Input: part model. Units: mm. Frame: model coordinates. Face numbers are marked on the shaded views. A direction names the side the tool comes from. Give positions to 0.01 mm unless a question says otherwise; leave off trailing zeros. Loops run counter-clockwise (first coordinate to the right, second up) from the corner with the lowest first, then second, coordinate; pieces in that order, holes last. Notation, with made-up numbers: (-32, -25.5) - (10, -25.5) arc R32 cw to (10, 0.5) - close; hole circle Ø5 at (51.25, -22.75). An arc over 180 degrees is marked (long way). Answer as a JSON object with one key per item and string values.
from build123d import *

# Parameters (mm, degrees)
SKETCH1_W           = 26.35
SKETCH1_H           = 50
SKETCH1_W_2         = 20
SKETCH1_H_2         = 43.65
BOSS_EXTRUDE1_DEPTH = 35
SKETCH2_W           = 26.35
SKETCH2_H           = 50
BOSS_EXTRUDE2_DEPTH = 3.175
BOSS_EXTRUDE3_DEPTH = 5
FILLET1_R           = 4
SKETCH6_W           = 10
SKETCH6_H           = 5
CUT_EXTRUDE3_DEPTH  = 3.175
SKETCH8_R           = 3.05
CUT_EXTRUDE5_DEPTH  = 2.7
BOSS_EXTRUDE4_START = -3.175
SKETCH9_W           = 6
SKETCH9_H           = 4
BOSS_EXTRUDE4_DEPTH = 12.5
SKETCH10_R          = 1
CUT_EXTRUDE6_DEPTH  = 15.675


with BuildPart() as part:
    # Sketch1 → Boss-Extrude1 (new body)
    with BuildSketch(Plane(origin=(0, 0, 0), x_dir=(1, 0, 0), z_dir=(0, 1, 0))):
        Rectangle(SKETCH1_W, SKETCH1_H)
        Rectangle(SKETCH1_W_2, SKETCH1_H_2, mode=Mode.SUBTRACT)
    extrude(amount=BOSS_EXTRUDE1_DEPTH)

    # Sketch2 → Boss-Extrude2 (add)
    with BuildSketch(Plane(origin=(0, 35, 0), x_dir=(1, 0, 0), z_dir=(0, 1, 0))):
        Rectangle(SKETCH2_W, SKETCH2_H)
    extrude(amount=BOSS_EXTRUDE2_DEPTH)

    # Sketch4 → Boss-Extrude3 (add)
    with BuildSketch(Plane.XZ):
        with BuildLine():
            Line((-8.6, -20), (-8.6, -21.825))
            Line((-8.6, -21.825), (-1.4, -21.825))
            Line((-1.4, -21.825), (-1.4, -20))
            ThreePointArc((-1.4, -20), (-5, -16.4), (-8.6, -20))
        make_face()
        with BuildLine():
            Line((-8.6, 21.825), (-1.4, 21.825))
            Line((-1.4, 21.825), (-1.4, 20))
            ThreePointArc((-1.4, 20), (-5, 16.4), (-8.6, 20))
            Line((-8.6, 20), (-8.6, 21.825))
        make_face()
    extrude(amount=-BOSS_EXTRUDE3_DEPTH)

    # Fillet1
    fillet1_edges = [part.edges().sort_by_distance(p)[0] for p in [
        (-13.175, 38.175, 0),
        (0, 38.175, 25),
        (13.175, 38.175, 0),
        (0, 38.175, -25),
        (13.175, 19.0875, 25),
        (-13.175, 19.0875, 25),
        (-13.175, 19.0875, -25),
        (13.175, 19.0875, -25),
    ]]
    fillet(fillet1_edges, radius=FILLET1_R)

    # Sketch6 → Cut-Extrude3 (cut)
    with BuildSketch(Plane.ZY.offset(13.175)):
        with Locations((0, 20.675)):
            Rectangle(SKETCH6_W, SKETCH6_H)
    extrude(amount=-CUT_EXTRUDE3_DEPTH, mode=Mode.SUBTRACT)

    # Sketch8 → Cut-Extrude5 (cut)
    with BuildSketch(Plane.XZ):
        with Locations(Location((-5, -20, 0), (0, 0, 270))):
            Circle(SKETCH8_R)
        with Locations(Location((-5, 20, 0), (0, 0, 270))):
            Circle(SKETCH8_R)
    extrude(amount=-CUT_EXTRUDE5_DEPTH, mode=Mode.SUBTRACT)

    # Sketch9 → Boss-Extrude4 (add)
    with BuildSketch(Plane(origin=(13.175, 0, 0), x_dir=(0, 0, -1), z_dir=(1, 0, 0)).offset(BOSS_EXTRUDE4_START)):
        with Locations((19.5, 9.6)):
            Rectangle(SKETCH9_W, SKETCH9_H)
        with Locations((-9.25, 9.6)):
            Rectangle(SKETCH9_W, SKETCH9_H)
    extrude(amount=-BOSS_EXTRUDE4_DEPTH)

    # Sketch10 → Cut-Extrude6 (cut)
    with BuildSketch(Plane.XZ.offset(-7.6)):
        with Locations(Location((3.75, 8.575, 0), (0, 0, 270))):
            Circle(SKETCH10_R)
        with Locations(Location((3.75, -18.825, 0), (0, 0, 270))):
            Circle(SKETCH10_R)
    extrude(amount=-CUT_EXTRUDE6_DEPTH, mode=Mode.SUBTRACT)


solid = part.part
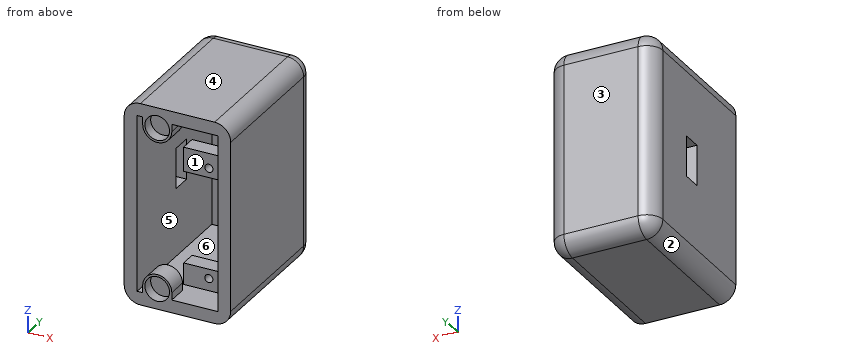
Item 1: Cut plane D-D (x = 3.75). Return loops of the section in (y, z) (3 decimals), then the cut area to 3 significant figures.
Geometry check:
{"outline": "(0, -25) - (34.175, -25) arc R4 ccw to (38.175, -21) - (38.175, 21) arc R4 ccw to (34.175, 25) - (0, 25) - (0, 21.825) - (35, 21.825) - (35, -21.825) - (11.6, -21.825) - (11.6, -19.825) - (7.6, -19.825) - (7.6, -21.825) - (0, -21.825) - close; (7.6, -17.825) - (11.6, -17.825) - (11.6, -16.5) - (7.6, -16.5) - close; (7.6, 6.25) - (11.6, 6.25) - (11.6, 7.575) - (7.6, 7.575) - close; (7.6, 9.575) - (11.6, 9.575) - (11.6, 12.25) - (7.6, 12.25) - close", "area": "403 mm2"}
Item 2: Cut plane C-C (z = 1). Return loops of the section in (x, y) (3 decimals).
Geometry check:
{"outline": "(-13.175, 0) - (-10, 0) - (-10, 18.175) - (-13.175, 18.175) - close; (-13.175, 23.175) - (-10, 23.175) - (-10, 35) - (10, 35) - (10, 0) - (13.175, 0) - (13.175, 34.175) arc R4 ccw to (9.175, 38.175) - (-9.175, 38.175) arc R4 ccw to (-13.175, 34.175) - close"}
Item 3: Access query for the marked faces 4, 5 and 6. Directions: +Z, -Z, +X, -X, +Y, -Y. A direction counts if a zero-diameter tool reaches every point of the face in a straight line with its end or side. Return the directions, or none.
Geometry check:
{"face 4": "+Z, +X, -X, +Y, -Y", "face 5": "-Y", "face 6": "none"}
Item 4: Cut plane A-A (x = 7.25). Return loops of the section in (y, z) (3 decimals), then the cut area to 3 significant figures.
Geometry check:
{"outline": "(0, -25) - (34.175, -25) arc R4 ccw to (38.175, -21) - (38.175, 21) arc R4 ccw to (34.175, 25) - (0, 25) - (0, 21.825) - (35, 21.825) - (35, -21.825) - (11.6, -21.825) - (11.6, -16.5) - (7.6, -16.5) - (7.6, -21.825) - (0, -21.825) - close; (7.6, 6.25) - (11.6, 6.25) - (11.6, 12.25) - (7.6, 12.25) - close", "area": "419 mm2"}
Item 5: Contact query for flat-ended pins moving along their axis: P1, Ø1.8, axis at x = -5.5, z = -19.5, coming from the -Y side; P2, Ø1.8, axis at x = 3.75, z = -18.825, coming from the -Y side; P3, Ø2.5, axis at x = -11.5, y = 19.5, coming from the +Z side. Output: stop coordinate, or through.
Geometry check:
{"P1": "stops at y = 2.7", "P2": "stops at y = 35", "P3": "stops at z = 24.85"}
Item 6: Material intervals for line 1 (X direction, y = 0.8, z = 20) (3 decimals); line 2 (X direction, y = 7, z = -14.5) (3 decimals); line 3 (Z direction, x = -1, y = 17.5) (3 decimals), sorted ascending. Write a range as [from, to].
Geometry check:
{"line 1": "x = [-13.175, -10], [-8.6, -8.05], [-1.95, -1.4], [10, 13.175]", "line 2": "x = [-13.175, -10], [10, 13.175]", "line 3": "z = [-25, -21.825], [21.825, 25]"}
Item 7: Mould query, pull axis Z, two halves, no side actions, for the marked faces 1, 2 and 3. Classes: released by +Z, released by -Z, zero draft, split by the parting line, or undercut.
Geometry check:
{"face 1": "undercut", "face 2": "released by -Z", "face 3": "zero draft"}
Item 8: Cut plane B-B (y = 6). Return loops of the section in (x, z) (3 decimals).
Geometry check:
{"outline": "(-13.175, -21) arc R4 ccw to (-9.175, -25) - (9.175, -25) arc R4 ccw to (13.175, -21) - (13.175, 21) arc R4 ccw to (9.175, 25) - (-9.175, 25) arc R4 ccw to (-13.175, 21) - close; hole (-10, -21.825) - (10, -21.825) - (10, 21.825) - (-10, 21.825) - close"}
